Verification items for the finished model (mm, model axes). A direction names the side the tool comes from. Coordinates: 2 decimals unless noted, no trailing zeros. Write each loop counter-clockwise with the first axis right and the second up, starting at its lowest first coordinate (ties: lowest second). Pieces come first, ordered by that corner, then holes. Notation, with made-up numbers: (89, 51.5) -> (140, 51.5) arc R29 ccw to (140, 78.5) -> close; hole circle Ø1 at (-10, 87.5). An arc over 180 degrees is marked (long way). Answer in a Markdown table with one row per item.
Autodesk Inventor part; units mm, degrees
ref_plane "YZ Plane" through (0, 0, 0) normal (1, 0, 0) x (0, 1, 0)
ref_plane "XZ Plane" through (0, 0, 0) normal (0, 1, 0) x (-1, 0, 0)
ref_plane "XY Plane" through (0, 0, 0) normal (0, 0, 1) x (1, 0, 0)
sketch "Sketch1" plane through (0, 0, 0) normal (0, 0, 1) x (1, 0, 0)
  line L0 (0, 4) -> (0, 0)
  line L1 (0, 0) -> (125, 0)
  line L2 (0, 4) -> (57, 23.5)
  line L3 (103, 14.5) -> (103, 8)
  line L4 (103, 8) -> (73, 8)
  line L5 (73, 8) -> (73, 14.5)
  line L6 (125, 14.5) -> (121, 14.5)
  line L7 (121, 14.5) -> (121, 8)
  line L8 (121, 8) -> (125, 8)
  line L9 (125, 0) -> (125, 8)
  line L10 (125, 14.5) -> (125, 23.5)
  line L11 (81, 23.5) -> (81, 14.5)
  line L12 (92, 14.5) -> (92, 23.5)
  line L13 (73, 14.5) -> (81, 14.5)
  line L14 (92, 14.5) -> (103, 14.5)
  line L15 (81, 14.5) -> (92, 14.5) construction
  circle A0 centre (86.5, 19.599) radius 7.5 construction
  circle A1 centre (86.5, 19.599) radius 4 construction
  line L16 (113.5, 21.9084) -> (113.5, 17.2896)
  line L17 (113.5, 17.2896) -> (109.5, 14.9802)
  line L18 (109.5, 14.9802) -> (105.5, 17.2896)
  line L19 (105.5, 17.2896) -> (105.5, 21.9084)
  line L20 (105.5, 21.9084) -> (109.5, 24.2178)
  line L21 (109.5, 24.2178) -> (113.5, 21.9084)
  circle A2 centre (109.5, 19.599) radius 2.5 construction
  line L22 (103.5, 23.5) -> (103.5, 29.5)
  line L23 (105.5, 31.5) -> (113.5, 31.5)
  line L24 (115.5, 29.5) -> (115.5, 23.5)
  arc A3 (105.5, 31.5) -> (103.5, 29.5) centre (105.5, 29.5) ccw
  arc A4 (115.5, 29.5) -> (113.5, 31.5) centre (113.5, 29.5) ccw
  line L25 (125, 23.5) -> (115.5, 23.5)
  line L26 (103.5, 23.5) -> (92, 23.5)
  circle A5 centre (99.5, 19) radius 4.5 construction
  circle A6 centre (119.5, 19) radius 4.5 construction
  circle A7 centre (99.5, 19) radius 2.25
  circle A8 centre (119.5, 19) radius 2.25
  line L27 (67, 23.5) -> (67, 29.5)
  line L28 (69, 31.5) -> (73, 31.5)
  line L29 (75, 29.5) -> (75, 23.5)
  arc A9 (69, 31.5) -> (67, 29.5) centre (69, 29.5) ccw
  arc A10 (75, 29.5) -> (73, 31.5) centre (73, 29.5) ccw
  line L30 (81, 23.5) -> (75, 23.5)
  line L31 (67, 23.5) -> (57, 23.5)
  point P0 (81, 14.5)
  point P1 (92, 14.5)
  point P2 (86.5, 14.5)
  point P3 (125, 19)
  point P4 (109.5, 31.5)
  dimension "d0" = 8
  dimension "d2" = 6.5
  dimension "d3" = 4
  dimension "d4" = 15
  dimension "d5" = 8
  dimension "d6" = 9
  dimension "d7" = 11
  dimension "d8" = 11
  dimension "d9" = 8
  dimension "d10" = 5
  dimension "d11" = 2
  dimension "d12" = 12
  dimension "d13" = 9
  dimension "d14" = 9
  dimension "d15" = 10
  dimension "d16" = 10
  dimension "d17" = 4.5
  dimension "d18" = 4.5
  dimension "d19" = 13
  dimension "d20" = 5.5
  dimension "d21" = 18
  dimension "d22" = 2
  dimension "d23" = 8
  dimension "d24" = 6
  dimension "d25" = 10
  dimension "d27" = 30
  dimension "d28" = 4
  dimension "d30" = 8
  dimension "d31" = 125
extrude "Extrusion1" add sketch "Sketch1" along normal blind 6.5
sketch "Sketch2" plane through (0, 0, 6.5) normal (0, 0, 1) x (1, 0, 0)
  line L0 (0, 4) -> (0, 0)
  line L1 (0, 0) -> (125, 0)
  line L2 (6, 0) -> (14, 0)
  line L3 (14, 0) -> (14, -4.5)
  line L4 (12, -6.5) -> (8, -6.5)
  line L5 (6, -4.5) -> (6, 0)
  line L6 (57, 0) -> (65, 0)
  line L7 (65, 0) -> (65, -4.5)
  line L8 (63, -6.5) -> (59, -6.5)
  line L9 (57, -4.5) -> (57, 0)
  line L10 (85, 0) -> (93, 0)
  line L11 (93, 0) -> (93, -4.5)
  line L12 (91, -6.5) -> (87, -6.5)
  line L13 (85, -4.5) -> (85, 0)
  line L14 (113, 0) -> (121, 0)
  line L15 (121, 0) -> (121, -4.5)
  line L16 (119, -6.5) -> (115, -6.5)
  line L17 (113, -4.5) -> (113, 0)
  arc A0 (6, -4.5) -> (8, -6.5) centre (8, -4.5) ccw
  arc A1 (12, -6.5) -> (14, -4.5) centre (12, -4.5) ccw
  arc A2 (57, -4.5) -> (59, -6.5) centre (59, -4.5) ccw
  arc A3 (63, -6.5) -> (65, -4.5) centre (63, -4.5) ccw
  arc A4 (85, -4.5) -> (87, -6.5) centre (87, -4.5) ccw
  arc A5 (91, -6.5) -> (93, -4.5) centre (91, -4.5) ccw
  arc A6 (113, -4.5) -> (115, -6.5) centre (115, -4.5) ccw
  arc A7 (119, -6.5) -> (121, -4.5) centre (119, -4.5) ccw
  dimension "d34" = 2
  dimension "d35" = 8
  dimension "d36" = 8
  dimension "d37" = 8
  dimension "d38" = 8
  dimension "d39" = 6.5
  dimension "d40" = 6
  dimension "d41" = 43
  dimension "d42" = 20
  dimension "d43" = 20
extrude "Extrusion2" add sketch "Sketch2" against normal blind 6.5
sketch "Sketch3" plane through (0, 0, 6.5) normal (0, 0, 1) x (1, 0, 0)
  line L0 (0, 4) -> (0, 0)
  line L1 (14, 0) -> (57, 0)
  line L2 (30, 0) -> (40, 0)
  line L3 (40, 0) -> (40, 5)
  line L4 (39, 6) -> (31, 6)
  line L5 (30, 5) -> (30, 0)
  arc A0 (31, 6) -> (30, 5) centre (31, 5) ccw
  arc A1 (40, 5) -> (39, 6) centre (39, 5) ccw
  point P0 (35, 6)
  dimension "d46" = 1
  dimension "d47" = 10
  dimension "d48" = 6
  dimension "d49" = 35
extrude "Extrusion3" cut sketch "Sketch3" against normal through all
properties part number "x_motor_wall_lower" material "Plywood, Finish"
1. Access from +Z, -Z, +X, -X, +Y, -Y to the whole of each face (thin tool, end or side, straight path). Record for faces 1 (the face through (85.57, -5.9, 3.3)), 2 (the face through (123, 0, 3)), 3 (the face through (75, 27, 3)), 4 (the face through (62, 23.5, 3)).
Findings below:
| item | result |
|---|---|
| face 1 | +Z, -Z, -Y |
| face 2 | +Z, -Z, +X, -Y |
| face 3 | +Z, -Z, +Y |
| face 4 | +Z, -Z, -X, +Y |
2. Sectioned sample at B-B, the plane x = 99.5. Record the cut outline in (y, z), and give its area (4 significant figures).
Findings below:
| item | result |
|---|---|
| outline | (0, 0) -> (8, 0) -> (8, 6.5) -> (0, 6.5) -> close; (14.5, 0) -> (16.75, 0) -> (16.75, 6.5) -> (14.5, 6.5) -> close; (21.25, 0) -> (23.5, 0) -> (23.5, 6.5) -> (21.25, 6.5) -> close |
| area | 81.25 mm² |
3. Sectioned sample at C-C, the plane y = 19. Record the cut outline in (x, z), and give its area (4 significant figures).
Findings below:
| item | result |
|---|---|
| outline | (43.85, 0) -> (81, 0) -> (81, 6.5) -> (43.85, 6.5) -> close; (92, 0) -> (97.25, 0) -> (97.25, 6.5) -> (92, 6.5) -> close; (101.75, 0) -> (105.5, 0) -> (105.5, 6.5) -> (101.75, 6.5) -> close; (113.5, 0) -> (117.25, 0) -> (117.25, 6.5) -> (113.5, 6.5) -> close; (121.75, 0) -> (125, 0) -> (125, 6.5) -> (121.75, 6.5) -> close |
| area | 345.5 mm² |
4. Sectioned sample at A-A, the plane y = -3. Record the cut outline in (x, z).
Findings below:
| item | result |
|---|---|
| outline | (6, 0) -> (14, 0) -> (14, 6.5) -> (6, 6.5) -> close; (57, 0) -> (65, 0) -> (65, 6.5) -> (57, 6.5) -> close; (85, 0) -> (93, 0) -> (93, 6.5) -> (85, 6.5) -> close; (113, 0) -> (121, 0) -> (121, 6.5) -> (113, 6.5) -> close |
5. Release check for a two-part mould opening along Y. For faces 5 (the face through (123, 14.5, 3)), 6 (the face through (125, 4, 3)), 7 (the face through (64.4, -5.93, 3.3)) record: released by +Y, released by -Y, zero draft, split by the parting line, or undercut.
Findings below:
| item | result |
|---|---|
| face 5 | undercut |
| face 6 | zero draft |
| face 7 | released by -Y |
6. Material ranges on probe 1 along Y at (x, z) = (99.5, 2.25); probe 2 along Y at (x, z) = (95.5, 1.5); probe 3 along X at (y, z) = (24.5, 3.75), recorded low to high. Write a range as from..to.
Findings below:
| item | result |
|---|---|
| probe 1 | y = 0..8, 14.5..16.75, 21.25..23.5 |
| probe 2 | y = 0..8, 14.5..23.5 |
| probe 3 | x = 67..75, 103.5..115.5 |
7. Go/stop test with flat-tipped pins: pin 1 (2 mm diameter, centred on y = -2, z = 4.5, fed in from +X); pin 2 (2 mm diameter, centred on y = -1.5, z = 4.5, fed in from -X); pin 3 (1 mm diameter, centred on x = 27.5, z = 1.5, fed in from -Y). Record where each tip stops, or that it passes through.
Findings below:
| item | result |
|---|---|
| pin 1 | stops at x = 121 |
| pin 2 | stops at x = 6 |
| pin 3 | stops at y = 0 |
8. Sectioned sample at D-D, the plane z = 5.5. Count the separate pieces of the cut face and the enclosed holes in it, and give its area (3 significant figures).
Findings below:
| item | result |
|---|---|
| separate pieces | 1 |
| enclosed holes | 3 |
| area | 2,270 mm² |
